```python
from build123d import *

# Parameters (mm, degrees)
ESQUISSE1_W        = 65
ESQUISSE1_H        = 96
ESQUISSE1_R        = 1.5
ESQUISSE1_W_2      = 55
ESQUISSE1_H_2      = 8
ESQUISSE1_W_3      = 5
ESQUISSE1_H_3      = 5
BOSS_EXTRU_1_DEPTH = 5
CONG_1_R           = 2


with BuildPart() as part:
    # Esquisse1 → Boss.-Extru.1 (new body)
    with BuildSketch(Plane.XY):
        with Locations((-12.5, 0)):
            Rectangle(ESQUISSE1_W, ESQUISSE1_H)
        with Locations((0, 21.5)):
            Circle(ESQUISSE1_R, mode=Mode.SUBTRACT)
        with Locations(Location((0, -21.5, 0), (0, 0, 90))):
            Circle(ESQUISSE1_R, mode=Mode.SUBTRACT)
        with Locations(Location((-25, 21.5, 0), (0, 0, 180))):
            Circle(ESQUISSE1_R, mode=Mode.SUBTRACT)
        with Locations((-25, -21.5)):
            Circle(ESQUISSE1_R, mode=Mode.SUBTRACT)
        with Locations((-12.5, -36)):
            Rectangle(ESQUISSE1_W_2, ESQUISSE1_H_2, mode=Mode.SUBTRACT)
        with Locations((-12.5, 36)):
            Rectangle(ESQUISSE1_W_2, ESQUISSE1_H_2, mode=Mode.SUBTRACT)
        with Locations((-7.5, 21.5)):
            Rectangle(ESQUISSE1_W_3, ESQUISSE1_H_3, mode=Mode.SUBTRACT)
        with Locations((7.5, 21.5)):
            Rectangle(ESQUISSE1_W_3, ESQUISSE1_H_3, mode=Mode.SUBTRACT)
        with Locations((-7.5, -21.5)):
            Rectangle(ESQUISSE1_W_3, ESQUISSE1_H_3, mode=Mode.SUBTRACT)
        with Locations((7.5, -21.5)):
            Rectangle(ESQUISSE1_W_3, ESQUISSE1_H_3, mode=Mode.SUBTRACT)
        with Locations((-17.5, 21.5)):
            Rectangle(ESQUISSE1_W_3, ESQUISSE1_H_3, mode=Mode.SUBTRACT)
        with Locations((-32.5, 21.5)):
            Rectangle(ESQUISSE1_W_3, ESQUISSE1_H_3, mode=Mode.SUBTRACT)
        with Locations((-17.5, -21.5)):
            Rectangle(ESQUISSE1_W_3, ESQUISSE1_H_3, mode=Mode.SUBTRACT)
        with Locations((-32.5, -21.5)):
            Rectangle(ESQUISSE1_W_3, ESQUISSE1_H_3, mode=Mode.SUBTRACT)
    extrude(amount=BOSS_EXTRU_1_DEPTH)

    # Congé1
    cong_1_edges = [part.edges().sort_by_distance(p)[0] for p in [
        (-40, 40, 2.5),
        (-40, 32, 2.5),
        (15, 32, 2.5),
        (15, 40, 2.5),
        (-40, -40, 2.5),
        (15, -40, 2.5),
        (15, -32, 2.5),
        (-40, -32, 2.5),
        (-45, -48, 2.5),
        (-45, 48, 2.5),
        (20, 48, 2.5),
        (20, -48, 2.5),
    ]]
    fillet(cong_1_edges, radius=CONG_1_R)


solid = part.part
```
Part model, mm, in its own coordinate system. Round coordinates to 2 decimals unless told otherwise and drop trailing zeros. Write each loop counter-clockwise with the first axis right and the second up, starting at its lowest first coordinate (ties: lowest second). Pieces come first, ordered by that corner, then holes. Notation, with made-up numbers: M 30,22 L 37,22 A27 ccw 37,60 Z; hole C -5,48 d6. An arc over 180 degrees is marked long. Answer as CSV lines item,"result". Start each with the question number.
1) Drill centre lines: L1, parallel to Y at x = -25, z = 1.4; L2, parallel to Y at x = -18.5, z = 1.45; L3, parallel to Y at x = -2, z = 2.4. Where is each one in solid material? Low to high.
2) Band-saw the part on C-C (x = -21). List the corners of the cut face in (y, z), then the cut area to 3 significant figures.
3) Band-saw the part on D-D (z = 2.65). Count the separate pieces of the cut face and the enclosed holes in it, then the cut area to 3 significant figures.
4) Drop flat-ended pins along their axis: pin 1 (5 mm diameter, centred on x = -23.5, y = 16, fed in from -Z); pin 2 (2.5 mm diameter, centred on x = 0, y = 21.5, fed in from +Z). Give the stop position or say it passes through.
5) Band-saw the part on B-B (x = -7.5). List the corners of the cut face in (y, z), then the cut area to 3 significant figures.
6) Band-saw the part on A-A (y = 21.5). List the corners of the cut face in (x, z), then the cut area to 3 significant figures.
Worked out:
1,L1,"-48 to -40, -32 to -23, -20 to 20, 23 to 32, 40 to 48"
1,L2,"-48 to -40, -32 to -24, -19 to 19, 24 to 32, 40 to 48"
1,L3,"-48 to -40, -32 to 32, 40 to 48"
2,outline,"M -48,0 L -40,0 L -40,5 L -48,5 Z; M -32,0 L 32,0 L 32,5 L -32,5 Z; M 40,0 L 48,0 L 48,5 L 40,5 Z"
2,area,"400 mm²"
3,separate pieces,"1"
3,enclosed holes,"14"
3,area,"5,140 mm²"
4,pin 1,"z = 0"
4,pin 2,"through"
5,outline,"M -48,0 L -40,0 L -40,5 L -48,5 Z; M -32,0 L -24,0 L -24,5 L -32,5 Z; M -19,0 L 19,0 L 19,5 L -19,5 Z; M 24,0 L 32,0 L 32,5 L 24,5 Z; M 40,0 L 48,0 L 48,5 L 40,5 Z"
5,area,"350 mm²"
6,outline,"M -45,0 L -35,0 L -35,5 L -45,5 Z; M -30,0 L -26.5,0 L -26.5,5 L -30,5 Z; M -23.5,0 L -20,0 L -20,5 L -23.5,5 Z; M -15,0 L -10,0 L -10,5 L -15,5 Z; M -5,0 L -1.5,0 L -1.5,5 L -5,5 Z; M 1.5,0 L 5,0 L 5,5 L 1.5,5 Z; M 10,0 L 20,0 L 20,5 L 10,5 Z"
6,area,"195 mm²"
